Work out the finished part from the listing and answer in its coordinate system (mm). Face numbers are marked on the shaded views. A direction names the side the tool comes from. Round coordinates to 2 decimals unless told otherwise and drop trailing zeros. Write each loop counter-clockwise with the first axis right and the second up, starting at its lowest first coordinate (ties: lowest second). Pieces come first, ordered by that corner, then holes. Notation, with made-up numbers: (75, 24.25) - (83, 24.25) arc R19 ccw to (83, 39.25) - close; hole circle Ø6 at (48.5, 18.25). An arc over 180 degrees is marked (long way). Answer as a JSON object with one key per item and string values.
```python
from build123d import *

# Parameters (mm, degrees)
MAIN_DEPTH         = 10
SKETCH2_R          = 1.6
CUT_EXTRUDE1_DEPTH = 4


with BuildPart() as part:
    # Sketch1 → Main (new body, symmetric)
    with BuildSketch(Plane.XY):
        Polygon((0, 19.3), (0, -19.3), (3, -19.3), (3, -11.3), (8, -11.3), (8, -4.1), (6.7, -4.1), (4.5, -6.3), (3, -6.3), (3, 6.3), (4.5, 6.3), (6.7, 4.1), (8, 4.1), (8, 11.3), (3, 11.3), (3, 19.3), align=None)
    extrude(amount=MAIN_DEPTH, both=True)

    # Sketch2 → Cut-Extrude1 (cut, through all)
    with BuildSketch(Plane(origin=(3, 0, 0), x_dir=(0, 0, -1), z_dir=(1, 0, 0))):
        with Locations((0, 15.3)):
            Circle(SKETCH2_R)
        with Locations((0, -15.3)):
            Circle(SKETCH2_R)
    extrude(amount=-CUT_EXTRUDE1_DEPTH, mode=Mode.SUBTRACT)


solid = part.part
```
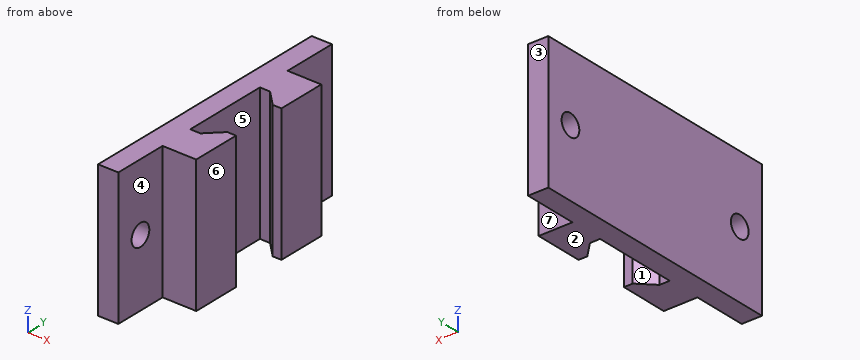
Item 1: A cutting plane is placed at A-A (x = 5.25). Write down the section's boundary in (y, z), and give its area (3 significant figures).
Results found:
{"outline": "(-11.3, -10) - (-5.55, -10) - (-5.55, 10) - (-11.3, 10) - close; (5.55, -10) - (11.3, -10) - (11.3, 10) - (5.55, 10) - close", "area": "230 mm²"}
Item 2: Consider line 1 along Y through (x, z) = (1.9, 0); line 2 along X through (y, z) = (1.5, -2); line 3 along Y through (x, z) = (6.5, -8.5). Determine where each line is inside the solid, lowest interval first.
Results found:
{"line 1": "-19.3 to -16.9, -13.7 to 13.7, 16.9 to 19.3", "line 2": "0 to 3", "line 3": "-11.3 to -4.3, 4.3 to 11.3"}
Item 3: A cutting plane is placed at D-D (x = 2.25). Write down the section's boundary in (y, z), and give its area (3 significant figures).
Results found:
{"outline": "(-19.3, -10) - (19.3, -10) - (19.3, 10) - (-19.3, 10) - close; hole circle Ø3.2 at (-15.3, 0); hole circle Ø3.2 at (15.3, 0)", "area": "756 mm²"}
Item 4: Determine the mould class of the marked faces 1, 2 and 3 for opening direction Y: pulls with the +Y half, pulls with the -Y half, needs draft (parallel to the pull), parting line crosses it, or undercut.
Results found:
{"face 1": "undercut", "face 2": "needs draft", "face 3": "pulls with the +Y half"}
Item 5: Each of these flat-tipped pins is pushed along its axis until it touches: P1, Ø6.5, axis at y = 17, z = -3, coming from the +X side; P2, Ø1, axis at x = 5.5, y = -12, coming from the -Z side; P3, Ø0.6, axis at x = 7, z = 1, coming from the -Y side; P4, Ø1, axis at x = 7.5, z = 2, coming from the +Y side. Where does it stop, or does it pass through?
Results found:
{"P1": "x = 3", "P2": "through", "P3": "y = -11.3", "P4": "y = 11.3"}
Item 6: For the marked faces 4, 5, 6 and 7, determine the directions among +Z, -Z, +X, -X, +Y, -Y from which every point of the face is accessible in a straight line to the end or side of a thin tool.
Results found:
{"face 4": "+Z, -Z, +X, -Y", "face 5": "+Z, -Z", "face 6": "+Z, -Z, +X, +Y, -Y", "face 7": "+Z, -Z, +X, +Y"}
Item 7: A cutting plane is placed at B-B (z = 0). Write down the section's boundary in (x, y), and give its area (3 significant figures).
Results found:
{"outline": "(0, -19.3) - (3, -19.3) - (3, -16.9) - (0, -16.9) - close; (0, -13.7) - (3, -13.7) - (3, -11.3) - (8, -11.3) - (8, -4.1) - (6.7, -4.1) - (4.5, -6.3) - (3, -6.3) - (3, 6.3) - (4.5, 6.3) - (6.7, 4.1) - (8, 4.1) - (8, 11.3) - (3, 11.3) - (3, 13.7) - (0, 13.7) - close; (0, 16.9) - (3, 16.9) - (3, 19.3) - (0, 19.3) - close", "area": "157 mm²"}
Item 8: A cutting plane is placed at C-C (y = -15.3). Write down the section's boundary in (x, z), and give its area (3 significant figures).
Results found:
{"outline": "(0, -10) - (3, -10) - (3, -1.6) - (0, -1.6) - close; (0, 1.6) - (3, 1.6) - (3, 10) - (0, 10) - close", "area": "50.4 mm²"}
